Check sheet for the modelled part. Datum: model origin and axes. Units: mm. Face numbers are marked on the shaded views. Round coordinates to 2 decimals unless told otherwise and drop trailing zeros. Write each loop counter-clockwise with the first axis right and the second up, starting at its lowest first coordinate (ties: lowest second). Pieces come first, ordered by that corner, then holes. Notation, with made-up numbers: (-36.5, -16) - (18.5, -16) arc R21 cw to (18.5, 2) - close; hole circle Ø10 at (74.5, 67). An arc over 180 degrees is marked (long way). Answer as a JSON object with one key per item and string values. Group by question number.
Item 1: Sectioned sample at B-B on z = 17. Record the boundary of the cut face in (x, y), plus the area to 3 significant figures.
Item 2: Thickness scan on line 1 (Z direction, x = -3.5, y = 0); line 2 (Y direction, x = 0, z = 14); line 3 (Y direction, x = -5.5, z = 3). Record the ranges inside material, lowest first.
Item 3: Gauge pin test, flat ends, axial feed: P1, Ø3, axis at x = 4.5, z = 15, coming from the -Y side; P2, Ø3, axis at x = 0, y = 0, coming from the +Z side; P3, Ø3, axis at x = -5.5, z = 15.5, coming from the +Y side; P4, Ø3, axis at x = -5, z = 2, coming from the -Y side. Record the tip position at first contact, or that the pin passes through.
Item 4: Sectioned sample at A-A on x = 0. Record the boundary of the cut face in (y, z), plus the area to 3 significant figures.
Item 5: Sectioned sample at D-D on z = 7.25. Record the boundary of the cut face in (x, y), plus the area to 3 significant figures.
Item 6: Release check for a two-part mould opening along Y. For the marked faces 1, 2 and 3 record: pulls with the +Y half, pulls with the -Y half, needs draft (parallel to the pull), parting line crosses it, or undercut.
Item 7: Sectioned sample at C-C on y = 0. Count the separate pieces of the cut face and the enclosed holes in it, plus the area to 3 significant figures.
Autodesk Inventor part; units mm, degrees
ref_plane "YZ Plane" through (0, 0, 0) normal (1, 0, 0) x (0, 1, 0)
ref_plane "XZ Plane" through (0, 0, 0) normal (0, 1, 0) x (-1, 0, 0)
ref_plane "XY Plane" through (0, 0, 0) normal (0, 0, 1) x (1, 0, 0)
sketch "Sketch1" plane through (0, 0, 0) normal (0, 0, 1) x (1, 0, 0)
  circle A0 centre (0, 0) radius 10
  dimension "d0" = 20
extrude "Extrusion1" add sketch "Sketch1" along normal blind 20
sketch "Sketch3" plane through (0, 0, 0) normal (0, 0, -1) x (-1, 0, 0)
  circle A0 centre (0, 0) radius 2.5
  dimension "d49" = 5
extrude "Extrusion3" cut sketch "Sketch3" against normal through all
sketch "Sketch4" plane through (0, 0, 0) normal (1, 0, 0) x (0, 1, 0)
  circle A0 centre (0, 3) radius 1.5
  line L0 (-10, 0) -> (10, 0)
  circle A1 centre (0, 17) radius 1.5
  line L1 (10, 20) -> (-10, 20)
  point P0 (0, 0)
  dimension "d9" = 3
  dimension "d10" = 3
  dimension "d11" = 3
  dimension "d12" = 3
sketch "Sketch5" plane through (0, 0, 20) normal (0, 0, 1) x (1, 0, 0)
  circle A0 centre (0, 0) radius 10
  line L0 (-8.5, -5.2678) -> (-8.5, 5.2678)
  dimension "d48" = 8.5
extrude "Extrusion5" cut sketch "Sketch5" against normal blind 21.25 contours L0 A0 picked at (-8.817, 1.0892)
mirror "Mirror1" about plane through (0, 0, 0) normal (1, 0, 0) of "Extrusion5"
chamfer "Chamfer1" distance 0.5 angle 45 2 edges at (2.5, 0, 0) (2.5, 0, 20)
chamfer "Chamfer2" distance 0.5 angle 45 8 edges at (0, 10, 20) (0, -10, 20) (8.5, 0, 20) (0, 10, 0) (0, -10, 0) (8.5, 0, 0) (-8.5, 0, 0) (-8.5, 0, 20)
hole "Hole1" at (0, 0, 17) at (0, 0, 3) direction (-1, 0, 0) diameter 3.5 end through all both
thread "Thread5"
thread "Thread6"
thread "Thread7"
thread "Thread8"
properties part number "КВ33.000.106 - Муфта" material "Aluminum 6061"
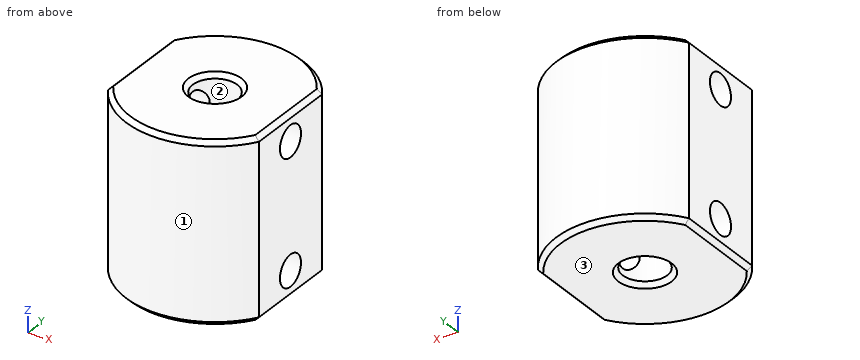
Completed:
{
 "1": {"outline": "(-8.5, -5.27) arc R10 ccw to (8.5, -5.27) - (8.5, -1.75) - (1.79, -1.75) arc R2.5 cw to (-1.79, -1.75) - (-8.5, -1.75) - close; (-8.5, 1.75) - (-1.79, 1.75) arc R2.5 cw to (1.79, 1.75) - (8.5, 1.75) - (8.5, 5.27) arc R10 ccw to (-8.5, 5.27) - close", "area": "230 mm²"},
 "2": {"line 1": "0 to 1.25, 4.75 to 15.25, 18.75 to 20", "line 2": "-10 to -2.5, 2.5 to 10", "line 3": "-8.35 to -1.75, 1.75 to 8.35"},
 "3": {"P1": "y = -9.54", "P2": "through", "P3": "y = 9.17", "P4": "y = -9.37"},
 "4": {"outline": "(-10, 0.5) - (-9.5, 0) - (-3, 0) - (-2.5, 0.5) - (-2.5, 19.5) - (-3, 20) - (-9.5, 20) - (-10, 19.5) - close; (2.5, 0.5) - (3, 0) - (9.5, 0) - (10, 0.5) - (10, 19.5) - (9.5, 20) - (3, 20) - (2.5, 19.5) - close", "area": "299 mm²"},
 "5": {"outline": "(-8.5, -5.27) arc R10 ccw to (8.5, -5.27) - (8.5, 5.27) arc R10 ccw to (-8.5, 5.27) - close; hole circle Ø5 at (0, 0)", "area": "273 mm²"},
 "6": {"face 1": "pulls with the -Y half", "face 2": "undercut", "face 3": "needs draft"},
 "7": {"separate pieces": "6", "enclosed holes": "0", "area": "155 mm²"}
}
